from build123d import *

# Parameters (mm, degrees)
SKETCH_1_W          = 12
SKETCH_1_H          = 12
EXTRUDE_1_DEPTH     = 3
SKETCH_2_W          = 4
SKETCH_2_H          = 4
CUT_EXTRUDE_1_DEPTH = 2
FILLET_1_R          = 1


with BuildPart() as part:
    # 스케치1 → 보스-돌출1 (new body)
    with BuildSketch(Plane.XY):
        Rectangle(SKETCH_1_W, SKETCH_1_H)
    extrude(amount=EXTRUDE_1_DEPTH)

    # 스케치2 → 컷-돌출1 (cut)
    with BuildSketch(Plane.XY.offset(3)):
        Rectangle(SKETCH_2_W, SKETCH_2_H)
    extrude(amount=-CUT_EXTRUDE_1_DEPTH, mode=Mode.SUBTRACT)

    # 필렛1
    fillet_1_edges = [part.edges().sort_by_distance(p)[0] for p in [
        (6, -6, 1.5),
        (-6, -6, 1.5),
        (-6, 6, 1.5),
        (6, 6, 1.5),
    ]]
    fillet(fillet_1_edges, radius=FILLET_1_R)


solid = part.part
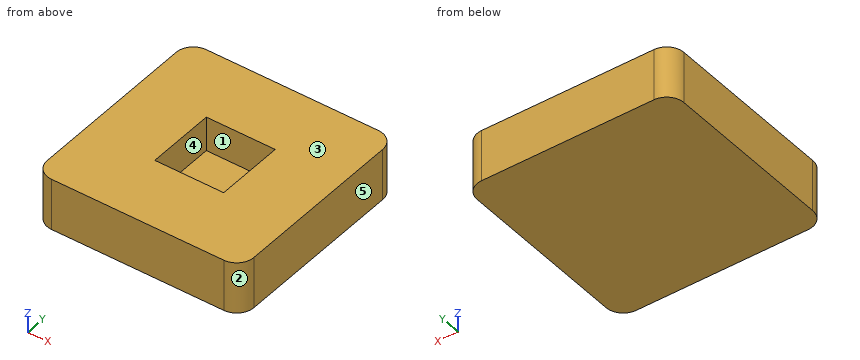
Verification items for the finished model (mm, model axes). Face numbers are marked on the shaded views. A direction names the side the tool comes from. Give positions to 0.01 mm unless a question says otherwise; leave off trailing zeros. Loops run counter-clockwise (first coordinate to the right, second up) from the corner with the lowest first, then second, coordinate; pieces in that order, holes last. Notation, with made-up numbers: (-38, 70) - (-11, 70) arc R8 cw to (-11, 79) - close; hole circle Ø3 at (54, -6). An arc over 180 degrees is marked (long way). Write item = value, one per line. Start each with the question number.
Q1. Tool access check on the marked faces 4 and 5. Record the directions out of +Z, -Z, +X, -X, +Y, -Y that give a thin tool (end or side, any length) a straight path to the whole face; none if there is none.
Q2. Cross-section at A-A, the plane z = 1.95. Enter the section's corners in (x, y), and give its area (3 significant figures).
Q3. Cross-section at B-B, the plane y = 1.25. Enter the section's corners in (x, z).
Q4. Thickness scan on line 1 (X direction, y = -1, z = 2.65); line 2 (Z direction, x = 0.75, y = 1.5). Record the ranges inside material, lowest first.
Q5. Mould release check, pull along Y, two halves, no side actions. Record for the marked faces 1, 2 and 3: released by +Y, released by -Y, zero draft, split by the parting line, or undercut.
Answer key:
q1.face_4 = +Z
q1.face_5 = +Z, -Z, +X, +Y, -Y
q2.outline = (-6, -5) arc R1 ccw to (-5, -6) - (5, -6) arc R1 ccw to (6, -5) - (6, 5) arc R1 ccw to (5, 6) - (-5, 6) arc R1 ccw to (-6, 5) - close; hole (-2, -2) - (2, -2) - (2, 2) - (-2, 2) - close
q2.area = 127 mm^2
q3.outline = (-6, 0) - (6, 0) - (6, 3) - (2, 3) - (2, 1) - (-2, 1) - (-2, 3) - (-6, 3) - close
q4.line_1 = -6 to -2, 2 to 6
q4.line_2 = 0 to 1
q5.face_1 = undercut
q5.face_2 = released by -Y
q5.face_3 = zero draft
